The model under review builds one solid part; all positions refer to its coordinate system, in mm. Face numbers are marked on the shaded views. A direction names the side the tool comes from. Coordinates: 2 decimals unless noted, no trailing zeros. Loops run counter-clockwise (first coordinate to the right, second up) from the corner with the lowest first, then second, coordinate; pieces in that order, holes last. Notation, with made-up numbers: (46.25, -20) - (60.25, -20) arc R26 ccw to (60.25, 5) - close; hole circle Ø4 at (30, 7.25). An arc over 180 degrees is marked (long way). Answer in a Markdown table with one row per item. Add a question column.
(1) Machinability: for the marked faces 1 and 2, which of the approach directions +Z, -Z, +X, -X, +Y, -Y give a long, thin tool a straight path to every point of the face, cutting with its end or side? Answer none if there is none.
(2) We need section B-B on y = 45.47. Write out the cut boundary in (x, z).
(3) For P1, Ø1.6, axis at x = 2, z = 1, coming from the +Y side; P2, Ø3.5, axis at x = 9.37, z = 12.5, coming from the +Y side; P3, Ø4, axis at y = 23, z = 7, coming from the +X side; P4, Ø5, axis at x = 15, z = -6.5, coming from the -Y side, all flat-tipped, find the tip position at first contact; note any pin that passes through.
(4) We need section A-A on x = 9.37. Write out the cut boundary in (y, z), plus the area to 3 significant figures.
(5) We need section C-C on z = -12.5. Write out the cut boundary in (x, y).
(6) We need section D-D on z = 1. Write out the cut boundary in (x, y), plus the area to 3 significant figures.
(7) For line 1 along Y through (x, z) = (1.85, 12); line 2 along X through (y, z) = (1.85, -12.5); line 3 along Z through (x, y) = (9, 2), list the stretches that pass through material, from the lowest coordinate up.
from build123d import *

# Parameters (mm, degrees)
BOSS_EXTRUDE1_DEPTH      = 17
BOSS_EXTRUDE1_DEPTH_BACK = 17
FILLET1_R                = 2.8
SKETCH4_R                = 1.5
CUT_EXTRUDE2_DEPTH       = 20
CUT_EXTRUDE3_REACH       = 73.68
SKETCH5_R                = 1.55
CUT_EXTRUDE4_DEPTH       = 72.67984375
CUT_EXTRUDE4_DEPTH_BACK  = 4
FILLET3_R                = 3
CUT_EXTRUDE5_DEPTH       = 5
SKETCH8_R                = 1.55
CUT_EXTRUDE8_DEPTH       = 10
CORTAR_EXTRUIR1_REACH    = 73.68
REDONDEO1_R              = 12


with BuildPart() as part:
    # Sketch1 → Boss-Extrude1 (new, two sides: drawn at the far end of the back side and taken through both)
    with BuildSketch(Plane.XY.offset(-BOSS_EXTRUDE1_DEPTH_BACK)):
        Polygon((0, 0), (0, 57), (3.2, 57), (3.2, 3.2), (40, 3.2), (40, 0), align=None)
    extrude(amount=BOSS_EXTRUDE1_DEPTH + BOSS_EXTRUDE1_DEPTH_BACK)

    # Fillet1
    fillet1_edges = [part.edges().sort_by_distance(p)[0] for p in [
        (3.2, 3.2, 0),
    ]]
    fillet(fillet1_edges, radius=FILLET1_R)

    # Sketch4 → Cut-Extrude2 (cut)
    with BuildSketch(Plane.XZ):
        with Locations(Location((9.37, -12.5, 0), (0, 0, 270))):
            Circle(SKETCH4_R)
        with Locations(Location((9.37, 12.5, 0), (0, 0, 270))):
            Circle(SKETCH4_R)
        with Locations(Location((34.37, -12.5, 0), (0, 0, 270))):
            Circle(SKETCH4_R)
        with Locations(Location((34.37, 12.5, 0), (0, 0, 270))):
            Circle(SKETCH4_R)
    extrude(amount=-CUT_EXTRUDE2_DEPTH, mode=Mode.SUBTRACT)

    # Sketch5 → Cut-Extrude3 (cut, up to next)
    with BuildSketch(Plane.XZ, mode=Mode.PRIVATE) as cut_extrude3_sk1:
        with Locations(Location((9.37, 12.5, 0), (0, 0, 270))):
            Circle(SKETCH5_R)
    cut_extrude3_tool1 = extrude(cut_extrude3_sk1.sketch, amount=-CUT_EXTRUDE3_REACH, mode=Mode.PRIVATE) & part.part
    # Sketch5 → Cut-Extrude3 (cut, up to next)
    with BuildSketch(Plane.XZ, mode=Mode.PRIVATE) as cut_extrude3_sk2:
        with Locations(Location((34.37, 12.5, 0), (0, 0, 270))):
            Circle(SKETCH5_R)
    cut_extrude3_tool2 = extrude(cut_extrude3_sk2.sketch, amount=-CUT_EXTRUDE3_REACH, mode=Mode.PRIVATE) & part.part
    # Sketch5 → Cut-Extrude3 (cut, up to next)
    with BuildSketch(Plane.XZ, mode=Mode.PRIVATE) as cut_extrude3_sk3:
        with Locations(Location((9.37, -12.5, 0), (0, 0, 270))):
            Circle(SKETCH5_R)
    cut_extrude3_tool3 = extrude(cut_extrude3_sk3.sketch, amount=-CUT_EXTRUDE3_REACH, mode=Mode.PRIVATE) & part.part
    # Sketch5 → Cut-Extrude3 (cut, up to next)
    with BuildSketch(Plane.XZ, mode=Mode.PRIVATE) as cut_extrude3_sk4:
        with Locations(Location((34.37, -12.5, 0), (0, 0, 270))):
            Circle(SKETCH5_R)
    cut_extrude3_tool4 = extrude(cut_extrude3_sk4.sketch, amount=-CUT_EXTRUDE3_REACH, mode=Mode.PRIVATE) & part.part
    add(cut_extrude3_tool1.solids().sort_by_distance((9.37, 0, 12.5))[0], mode=Mode.SUBTRACT)
    add(cut_extrude3_tool2.solids().sort_by_distance((34.37, 0, 12.5))[0], mode=Mode.SUBTRACT)
    add(cut_extrude3_tool3.solids().sort_by_distance((9.37, 0, -12.5))[0], mode=Mode.SUBTRACT)
    add(cut_extrude3_tool4.solids().sort_by_distance((34.37, 0, -12.5))[0], mode=Mode.SUBTRACT)

    # Sketch6 → Cut-Extrude4 (cut, two sides: drawn at the far end of the back side and taken through both)
    with BuildSketch(Plane.ZY.offset(-CUT_EXTRUDE4_DEPTH_BACK)):
        Polygon((7, 57), (-17, 57), (-17, 8), (7, 37.8), align=None)
    extrude(amount=CUT_EXTRUDE4_DEPTH + CUT_EXTRUDE4_DEPTH_BACK, mode=Mode.SUBTRACT)

    # Fillet3
    fillet3_edges = [part.edges().sort_by_distance(p)[0] for p in [
        (40, 1.6, 17),
        (40, 1.6, -17),
    ]]
    fillet(fillet3_edges, radius=FILLET3_R)

    # Sketch7 → Cut-Extrude5 (cut)
    with BuildSketch(Plane.ZY):
        Polygon((-7.454709153, 9), (7, 9), (7.028471746, 12.409902656), (7.004699048, 26.953765183), align=None)
    extrude(amount=-CUT_EXTRUDE5_DEPTH, mode=Mode.SUBTRACT)

    # Sketch8 → Cut-Extrude8 (cut)
    with BuildSketch(Plane.ZY):
        with Locations((12, 52.47)):
            Circle(SKETCH8_R)
        with Locations((12, 45.47)):
            Circle(SKETCH8_R)
    extrude(amount=-CUT_EXTRUDE8_DEPTH, mode=Mode.SUBTRACT)

    # Croquis1 → Cortar-Extruir1 (cut, up to next)
    with BuildSketch(Plane.ZY, mode=Mode.PRIVATE) as cortar_extruir1_sk1:
        Polygon((17, 20), (14, 21.732050808), (14, 38.267949192), (17, 40), align=None)
    cortar_extruir1_tool1 = extrude(cortar_extruir1_sk1.sketch, amount=-CORTAR_EXTRUIR1_REACH, mode=Mode.PRIVATE) & part.part
    add(cortar_extruir1_tool1.solids().sort_by_distance((0, 30, 15.547407))[0], mode=Mode.SUBTRACT)

    # Redondeo1
    redondeo1_edges = [part.edges().sort_by_distance(p)[0] for p in [
        (1.6, 37.8, 7),
    ]]
    fillet(redondeo1_edges, radius=REDONDEO1_R)


solid = part.part
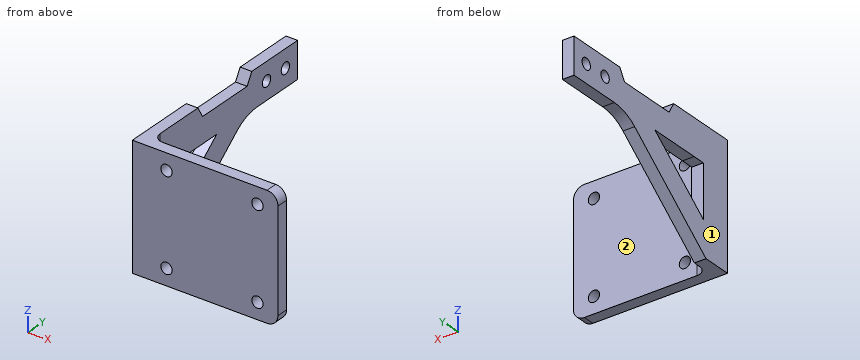
Outcome:
| question | item | result |
|---|---|---|
| 1 | face 1 | +Z, -Z, -X, +Y, -Y |
| 1 | face 2 | +Z, -Z, +X, +Y |
| 2 | outline | (0, 7) - (3.2, 7) - (3.2, 10.45) - (0, 10.45) - close; (0, 13.55) - (3.2, 13.55) - (3.2, 17) - (0, 17) - close |
| 3 | P1 | y = 31.34 |
| 3 | P2 | y = 3.2 |
| 3 | P3 | x = 3.2 |
| 3 | P4 | y = 0 |
| 4 | outline | (0, -17) - (3.2, -17) - (3.2, -14.05) - (0, -14.05) - close; (0, -10.95) - (3.2, -10.95) - (3.2, 10.95) - (0, 10.95) - close; (0, 14.05) - (3.2, 14.05) - (3.2, 17) - (0, 17) - close |
| 4 | area | 89.0 mm² |
| 5 | outline | (0, 0) - (7.82, 0) - (7.82, 3.2) - (6, 3.2) arc R2.8 cw to (3.2, 6) - (3.2, 13.59) - (0, 13.59) - close; (10.92, 0) - (32.82, 0) - (32.82, 3.2) - (10.92, 3.2) - close; (35.92, 0) - (40, 0) - (40, 3.2) - (35.92, 3.2) - close |
| 6 | outline | (0, 0) - (40, 0) - (40, 3.2) - (6, 3.2) arc R2.8 cw to (3.2, 6) - (3.2, 9) - (0, 9) - close; (0, 19.5) - (3.2, 19.5) - (3.2, 30.35) - (0, 30.35) - close |
| 6 | area | 183 mm² |
| 7 | line 1 | 0 to 43.92, 47.02 to 50.92, 54.02 to 57 |
| 7 | line 2 | 0 to 7.82, 10.92 to 32.82, 35.92 to 40 |
| 7 | line 3 | -17 to -14.01, -10.99 to 10.99, 14.01 to 17 |
